Source: CAD feature listing. Evaluate the final solid. Frame: model axes, mm. A direction names the side the tool comes from. Give positions to 0.01 mm unless a question says otherwise; leave off trailing zeros. Write each loop counter-clockwise with the first axis right and the second up, starting at its lowest first coordinate (ties: lowest second). Pieces come first, ordered by that corner, then holes. Notation, with made-up numbers: M 10.25,67.25 L 56.25,67.25 A7 ccw 56.25,80.25 Z; hole C 65,44 d4. An arc over 180 degrees is marked long. Use CSV: the item, a comma, the result in double quotes. Start each with the question number.
from build123d import *

# Parameters (mm, degrees)
EXTRUDE_1_DEPTH     = 5
SKETCH_2_R          = 13
CUT_EXTRUDE_1_DEPTH = 5
FILLET_1_R          = 5
HOLE_WIZARD_M3_1_D  = 3.4
CHAMFER1_SIZE       = 0.5


with BuildPart() as part:
    # 草图1 → 凸台-拉伸1 (new body)
    with BuildSketch(Plane(origin=(0, 0, 0), x_dir=(1, 0, 0), z_dir=(0, 1, 0))):
        with BuildLine():
            Line((45.228756555, 30), (64, 30))
            Line((64, 30), (64, 0))
            Line((64, 0), (45.228756555, 0))
            ThreePointArc((45.228756555, 0), (32, -5), (18.771243445, 0))
            Line((18.771243445, 0), (0, 0))
            Line((0, 0), (0, 30))
            Line((0, 30), (18.771243445, 30))
            ThreePointArc((18.771243445, 30), (32, 35), (45.228756555, 30))
        make_face()
    extrude(amount=EXTRUDE_1_DEPTH)

    # 草图2 → 切除-拉伸1 (cut)
    with BuildSketch(Plane(origin=(0, 5, 0), x_dir=(1, 0, 0), z_dir=(0, 1, 0))):
        with Locations((32, 15)):
            Circle(SKETCH_2_R)
    extrude(amount=-CUT_EXTRUDE_1_DEPTH, mode=Mode.SUBTRACT)

    # 圆角1
    fillet_1_edges = [part.edges().sort_by_distance(p)[0] for p in [
        (0, 2.5, -30),
        (18.771243445, 2.5, -30),
        (45.228756555, 2.5, -30),
        (64, 2.5, -30),
        (64, 2.5, 0),
        (0, 2.5, 0),
    ]]
    fillet(fillet_1_edges, radius=FILLET_1_R)

    # M3 间隙孔1 (through all)
    with Locations(Plane(origin=(0, 0, 0), x_dir=(-1, 0, 0), z_dir=(0, -1, 0))):
        with Locations((-56, 22.5), (-56, 12.5), (-8, 22.5), (-8, 12.5)):
            Hole(HOLE_WIZARD_M3_1_D / 2)

    # Chamfer1
    chamfer1_edges = [part.edges().sort_by_distance(p)[0] for p in [
        (19, 0, -15),
        (19, 5, -15),
    ]]
    chamfer(chamfer1_edges, length=CHAMFER1_SIZE)


solid = part.part
1. Section A-A on x = 32. Return loops of the section in (y, z), then the cut area to 3 significant figures.
2. Line query: probe 1 along Z at (x, y) = (56, 3.65); probe 2 along X at (y, z) = (2.55, -12.5); probe 3 along X at (y, z) = (2.55, -20). Output: solid intervals per line, ascending.
3. First-contact query: pin 1 (2.5 mm diameter, centred on x = 12.5, y = 1.5, fed in from -Z); pin 2 (2.5 mm diameter, centred on x = 56, z = -12.5, fed in from -Y); pin 3 (2.5 mm diameter, centred on x = 9, y = 3.5, fed in from +Z). Flat tips, straight axial feed; report the tip coordinate or a pass-through.
4. Pull-direction query (Z, two-part tool) for faces 6 (the cylindrical face through (32, 2, -35)), 7 (the cylindrical face through (7.779, 2.535, -24.186)), 8 (the flat face through (32, 0, -29)); classes: released by +Z, released by -Z, zero draft, split by the parting line, or undercut.
5. Section C-C on y = 1.2. Return loops of the section in (x, z), then the cut area to 3 significant figures.
6. Section D-D on z = -21.5. Give the number of separate pieces and of enclosed holes in the cut face, then the cut area to 3 significant figures.
7. Section B-B on x = 8. Return loops of the section in (y, z), then the cut area to 3 significant figures.
8. Access query for faces 1 (the flat face through (32, 5, -29)), 2 (the flat face through (53, 2, -30)), 3 (the flat face through (11, 2, -30)), 4 (the flat face through (12, 2, 0)), 5 (the flat face through (64, 2, -15)). Directions: +Z, -Z, +X, -X, +Y, -Y. A direction counts if a zero-diameter tool reaches every point of the face in a straight line with its end or side. Return the directions, or none.
Resolved:
1,outline,"M 0,-35 L 5,-35 L 5,-28.5 L 4.5,-28 L 0.5,-28 L 0,-28.5 Z; M 0,-1.5 L 0.5,-2 L 4.5,-2 L 5,-1.5 L 5,5 L 0,5 Z"
1,area,"69.5 mm2"
2,probe 1,"z = -30 to -24.2, -20.8 to -14.2, -10.8 to 0"
2,probe 2,"x = 0 to 6.3, 9.7 to 19.24, 44.76 to 54.3, 57.7 to 64"
2,probe 3,"x = 0 to 20, 44 to 64"
3,pin 1,"stops at z = -30"
3,pin 2,"passes through"
3,pin 3,"stops at z = 0"
4,face 6,"released by -Z"
4,face 7,"undercut"
4,face 8,"zero draft"
5,outline,"M 0,-25 A5 ccw 5,-30 L 17,-30 A5 cw 20,-31 A20 ccw 44,-31 A5 cw 47,-30 L 59,-30 A5 ccw 64,-25 L 64,-5 A5 ccw 59,0 L 45.23,0 A20 ccw 18.77,0 L 5,0 A5 ccw 0,-5 Z; hole C 8,-22.5 d3.4; hole C 8,-12.5 d3.4; hole C 32,-15 d26; hole C 56,-22.5 d3.4; hole C 56,-12.5 d3.4"
5,area,"1,510 mm2"
6,separate pieces,"4"
6,enclosed holes,"0"
6,area,"179 mm2"
7,outline,"M 0,-30 L 5,-30 L 5,-24.2 L 0,-24.2 Z; M 0,-20.8 L 5,-20.8 L 5,-14.2 L 0,-14.2 Z; M 0,-10.8 L 5,-10.8 L 5,0 L 0,0 Z"
7,area,"116 mm2"
8,face 1,"+Z, -Z, +X, -X, +Y"
8,face 2,"-Z, +X, +Y, -Y"
8,face 3,"-Z, -X, +Y, -Y"
8,face 4,"+Z, -X, +Y, -Y"
8,face 5,"+Z, -Z, +X, +Y, -Y"
